Source: CAD feature listing. Evaluate the final solid. Frame: model axes, mm. A direction names the side the tool comes from. Coordinates: 2 decimals unless noted, no trailing zeros. Order: outer loops, then holes, each group sorted by start corner. A loop starts at its lowest first (then second) coordinate and runs counter-clockwise, first axis right, second up. Notation, with made-up numbers: (51.5, 80) -> (76.5, 80) arc R26 cw to (76.5, 115) -> close; hole circle Ø3 at (89, 25). An arc over 180 degrees is marked (long way). Write each question's results on one line, items separated by ' | '. Start each with the question number.
Autodesk Fusion 360 part; units mm, degrees
sketch "Skizze1" plane through (0, 0, 0) normal (0, 0, 1) x (1, 0, 0)
  line L0 (0, 0) -> (15, 0)
  line L1 (15, 0) -> (15, -25)
  line L2 (15, -25) -> (0, -25)
  line L3 (0, -25) -> (0, 0)
extrude "Extrusion1" add sketch "Skizze1" along normal blind 5
sketch "Skizze2" plane through (0, 0, 5) normal (0, 0, 1) x (-1, 0, 0)
  line L0 (0, 25) -> (-15, 25)
  line L1 (-15, 25) -> (-15, 0)
  line L2 (-15, 0) -> (0, 0)
  line L3 (0, 0) -> (0, 25)
  line L4 (-5, 20) -> (-10, 20)
  line L5 (-10, 20) -> (-10, 25)
  line L6 (-10, 25) -> (-5, 25)
  line L7 (-5, 25) -> (-5, 20)
  dimension "d3" = 5
extrude "Extrusion2" add sketch "Skizze2" along normal blind 10 contours L0 L4 L5 L6 L7
sketch "Skizze3" plane through (0, -20, 0) normal (0, 1, 0) x (-1, 0, 0)
  line L0 (-10, 5) -> (-5, 5)
  line L1 (-5, 5) -> (-5, 15)
  line L2 (-5, 15) -> (-10, 15)
  line L3 (-10, 15) -> (-10, 5)
  line L4 (-10, 15) -> (-5, 15)
  line L5 (-5, 15) -> (-5, 10)
  line L6 (-5, 10) -> (-10, 10)
  line L7 (-10, 10) -> (-10, 15)
extrude "Extrusion3" add sketch "Skizze3" along normal blind 5 contours L1 L2 L3 L4 L5 L6 L7
hole "Bohrung1" at (7.5542, -5.0286, 5) direction (0, 0, -1) diameter 5 depth 15 tip angle 118
hole "Bohrung2" at (7.5, -11.7857, 5) direction (0, 0, -1) diameter 5 depth 15 tip angle 118
sketch "Skizze4" plane through (5, 0, 0) normal (-1, 0, 0) x (0, -1, 0)
  line L0 (20, 5) -> (25, 5)
  line L1 (25, 5) -> (25, 15)
  line L2 (25, 15) -> (15, 15)
  line L3 (15, 15) -> (15, 10)
  line L4 (15, 10) -> (20, 10)
  line L5 (20, 10) -> (20, 5)
  line L6 (20, 10) -> (15, 12.5)
  line L7 (15, 10) -> (20, 10)
extrude "Extrusion4" cut sketch "Skizze4" against normal blind 5 contours L3 L4 L6 L7
(1) Section A-A on y = -19.5. Return the cut outline in (x, z).
(2) Section C-C on y = -23. Return the cut outline in (x, z), then the cut area to 3 significant figures.
(3) Draft query along Y for faces 6 (the cylindrical face through (5.075, -4.703, 2.465)), 7 (the flat face through (7, -20, 7)), 8 (the flat face through (7, -20, 15)). Return one class per face: released by +Y, released by -Y, zero draft, split by the parting line, or undercut.
(4) Section B-B on x = 8.5. Return the cut outline in (y, z).
(5) Reachability of faces 1 (the flat face through (10, -21, 11)), 2 (the flat face through (8, -15, 14)), 3 (the flat face through (7, -18, 11)), 4 (the flat face through (0, -13, 2)), 5 (the flat face through (5, -21, 11)) from +Z, -Z, +X, -X, +Y, -Y: full face, straight path, thin tool, end or side. Return the list, or none.
(6) First-contact query: P1, Ø3, axis at x = 7.5, z = 14.5, coming from the +Y side; P2, Ø3, axis at y = -18, z = 12, coming from the +X side; P3, Ø3, axis at y = -20, z = 12, coming from the -X side; P4, Ø6, axis at y = -11, z = 7, coming from the -X side. Flat tips, straight axial feed; report the tip coordinate or a pass-through.
(7) Line query: L1, parallel to Y at x = 7.5, z = 2.3; L2, parallel to Y at x = 7.5, z = 5.75; L3, parallel to Z at x = 9.25, y = -14. Output: solid intervals per line, ascending.
(8) Section D-D on z = 5.5. Return the cut outline in (x, y), then the cut area to 3 significant figures.
Results list:
1) outline: (0, 0) -> (15, 0) -> (15, 5) -> (0, 5) -> close; (5, 10.25) -> (10, 10.25) -> (10, 15) -> (5, 15) -> close
2) outline: (0, 0) -> (15, 0) -> (15, 5) -> (10, 5) -> (10, 15) -> (5, 15) -> (5, 5) -> (0, 5) -> close | area: 125 mm²
3) face 6: undercut | face 7: released by +Y | face 8: zero draft
4) outline: (-25, 0) -> (-14.08, 0) -> (-14.08, 5) -> (-20, 5) -> (-20, 10) -> (-15, 12.5) -> (-15, 15) -> (-25, 15) -> close; (-9.49, 0) -> (-7.34, 0) -> (-7.34, 5) -> (-9.49, 5) -> close; (-2.71, 0) -> (0, 0) -> (0, 5) -> (-2.71, 5) -> close
5) face 1: +Z, +X, +Y, -Y | face 2: +Z, +X, -X, +Y | face 3: +X, -X, +Y | face 4: +Z, -Z, -X, +Y, -Y | face 5: +Z, -X, +Y, -Y
6) P1: stops at y = -15 | P2: stops at x = 10 | P3: stops at x = 5 | P4: stops at x = 0
7) L1: y = -25 to -14.29, -9.29 to -7.53, -2.53 to 0 | L2: y = -25 to -20 | L3: z = 0 to 5
8) outline: (5, -25) -> (10, -25) -> (10, -20) -> (5, -20) -> close | area: 25.0 mm²
